from build123d import *

# Parameters (mm, degrees)
F0_W     = 609.6
F0_H     = 304.8
F1_DEPTH = 76.2
F3_W     = 152.4
F3_H     = 152.4
F6_W     = 152.4
F6_H     = 152.4
F9_W     = 152.4
F9_H     = 152.4
F12_W    = 152.4
F12_H    = 152.4


with BuildPart() as f1:
    # F0 (on Front) → F1 (new body)
    with BuildSketch(Plane.XZ):
        Rectangle(F0_W, F0_H)
    extrude(amount=F1_DEPTH)

    # F3 (on face) → F5 section 0
    with BuildSketch(Plane.XZ.offset(76.2), mode=Mode.PRIVATE) as f5_s0:
        with Locations((-228.6, 76.2)):
            Rectangle(F3_W, F3_H)
    loft([f5_s0.sketch, Vertex(-228.6, -381, 76.2)])

    # F6 (on face) → F8 section 0
    with BuildSketch(Plane.XZ.offset(76.2), mode=Mode.PRIVATE) as f8_s0:
        with Locations((-76.2, 76.2)):
            Rectangle(F6_W, F6_H)
    loft([f8_s0.sketch, Vertex(-76.2, -381, 76.2)])

    # F9 (on face) → F11 section 0
    with BuildSketch(Plane.XZ.offset(76.2), mode=Mode.PRIVATE) as f11_s0:
        with Locations((-228.6, -76.2)):
            Rectangle(F9_W, F9_H)
    loft([f11_s0.sketch, Vertex(-228.6, -381, -76.2)])

    # F12 (on face) → F14 section 0
    with BuildSketch(Plane.XZ.offset(76.2), mode=Mode.PRIVATE) as f14_s0:
        with Locations((-76.2, -76.2)):
            Rectangle(F12_W, F12_H)
    loft([f14_s0.sketch, Vertex(-76.2, -381, -76.2)])

    # F15: F1 across plane


with BuildPart() as f1_1:
    add(f1.part)
    add(f1.part.mirror(Plane.YZ))


solid = f1_1.part
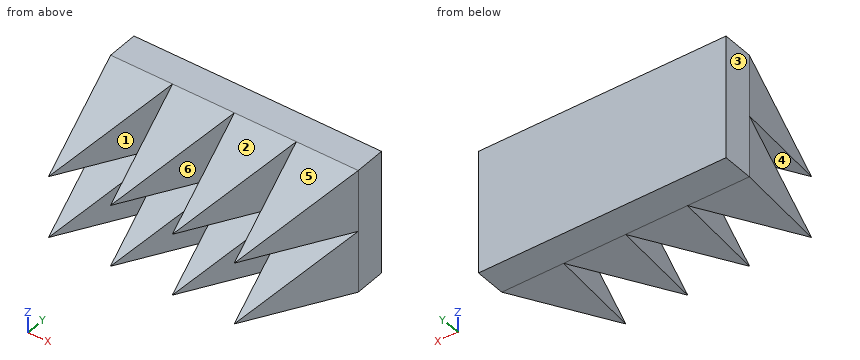
Verification items for the finished model (mm, model axes). Face numbers are marked on the shaded views. A direction names the side the tool comes from. Give positions to 0.01 mm unless a question says otherwise; leave off trailing zeros. Write each loop counter-clockwise with the first axis right and the second up, starting at its lowest first coordinate (ties: lowest second). Pieces come first, ordered by that corner, then holes.
(1) Cross-section at C-C (x = 211). Enter the section's corners in (y, z).
(2) Access from +Z, -Z, +X, -X, +Y, -Y to the whole of each face (thin tool, end or side, straight path). Record for the marked faces 4, 5 and 6.
(3) Cross-section at A-A (y = -234). State how many separate pieces and enclosed holes the cut face has, plus the area to 3 significant figures.
(4) Cross-section at B-B (z = 92). Enter the section's corners in (x, y), plus the area to 3 significant figures.
(5) Gauge pin test, flat ends, axial feed: pin 1 (8 mm diameter, centred on y = -262.5, z = -39.5, fed in from +X); pin 2 (4 mm diameter, centred on y = -167, z = 88.5, fed in from -X); pin 3 (5 mm diameter, centred on x = -78.5, y = -197, fed in from +Z) (3 decimals); pin 4 (1.5 mm diameter, centred on y = -79.5, z = -118, fed in from -X). Record the tip position at first contact, or that the pin passes through.
(6) Material ranges on line 1 (X direction, y = -235, z = 57); line 2 (X direction, y = -238, z = 92); line 3 (Z direction, x = -204, y = -114.5) (3 decimals), recorded low to high.
(7) Mould release check, pull along X, two halves, no side actions. Record for the marked faces 1, 2 and 3: +X half, -X half, draft (parallel to the pull), parting line (faces both ways), or undercut.
Worked out:
1. outline: (-310.6, -93.8) - (-76.2, -152.4) - (0, -152.4) - (0, 152.4) - (-76.2, 152.4) - (-310.6, 93.8) - (-310.6, 58.6) - (-76.2, 0) - (-310.6, -58.6) - close
2. face 4: +X, -X, -Y
2. face 5: +Z, +X, -X, -Y
2. face 6: +Z, -Z, -Y
3. separate pieces: 8
3. enclosed holes: 0
3. area: 43,200 mm2
4. outline: (-304.8, -76.2) - (-244.4, -317.8) - (-212.8, -317.8) - (-152.4, -76.2) - (-92, -317.8) - (-60.4, -317.8) - (0, -76.2) - (60.4, -317.8) - (92, -317.8) - (152.4, -76.2) - (212.8, -317.8) - (244.4, -317.8) - (304.8, -76.2) - (304.8, 0) - (-304.8, 0) - close
4. area: 135,000 mm2
5. pin 1: passes through
5. pin 2: stops at x = -282.6
5. pin 3: stops at z = 122.825
5. pin 4: stops at x = -304.16
6. line 1: x = -265.1 to -192.1, -112.7 to -39.7, 39.7 to 112.7, 192.1 to 265.1
6. line 2: x = -264.35 to -192.85, -111.95 to -40.45, 40.45 to 111.95, 192.85 to 264.35
6. line 3: z = -142.825 to -9.575, 9.575 to 142.825
7. face 1: undercut
7. face 2: draft
7. face 3: -X half
